from build123d import *

# Parameters (mm, degrees)
SKETCH1_W             = 35
SKETCH1_H             = 35
BOSS_EXTRUDE1_DEPTH   = 10
BOSS_EXTRUDE2_DEPTH   = 6
M10_CLEARANCE_HOLE1_D = 11
M6_CLEARANCE_HOLE1_D  = 6.6
MIRROR2_COPY_1_D      = 6.6


with BuildPart() as part:
    # Sketch1 → Boss-Extrude1 (new body)
    # profile 1 of 2: a face of its own
    with BuildSketch(Plane(origin=(0, 0, 0), x_dir=(1, 0, 0), z_dir=(0, 1, 0))):
        Rectangle(SKETCH1_W, SKETCH1_H)
        Polygon((-5.17766953, -12.5), (5.17766953, -12.5), (12.5, -5.17766953), (12.5, 5.17766953), (5.17766953, 12.5), (-5.17766953, 12.5), (-12.5, 5.17766953), (-12.5, -5.17766953), align=None, mode=Mode.SUBTRACT)
    # profile 2 of 2: a face of its own
    with BuildSketch(Plane(origin=(0, 0, 0), x_dir=(1, 0, 0), z_dir=(0, 1, 0))):
        Polygon((-12.5, -5.17766953), (-5.17766953, -12.5), (5.17766953, -12.5), (12.5, -5.17766953), (12.5, 5.17766953), (5.17766953, 12.5), (-5.17766953, 12.5), (-12.5, 5.17766953), align=None)
    extrude(amount=-BOSS_EXTRUDE1_DEPTH)

    # Sketch1_3 → Boss-Extrude2 (add)
    with BuildSketch(Plane(origin=(0, 0, 0), x_dir=(1, 0, 0), z_dir=(0, 1, 0))):
        Polygon((-12.5, -5.17766953), (-5.17766953, -12.5), (5.17766953, -12.5), (12.5, -5.17766953), (12.5, 5.17766953), (5.17766953, 12.5), (-5.17766953, 12.5), (-12.5, 5.17766953), align=None)
    extrude(amount=BOSS_EXTRUDE2_DEPTH)

    # M10 Clearance Hole1 (through all)
    with Locations(Plane(origin=(0, 6, 0), x_dir=(1, 0, 0), z_dir=(0, 1, 0))):
        with Locations((0, 0)):
            Hole(M10_CLEARANCE_HOLE1_D / 2)

    # M6 Clearance Hole1 (through all)
    with Locations(Plane(origin=(0, 0, 0), x_dir=(1, 0, 0), z_dir=(0, 1, 0))):
        with Locations((-12.5, 12.5)):
            m6_clearance_hole1 = Hole(M6_CLEARANCE_HOLE1_D / 2)

    # Mirror1: M6 Clearance Hole1 across plane
    add(m6_clearance_hole1.mirror(Plane(origin=(0, 0, 0), x_dir=(0, 0, 1), z_dir=(1, 0, 0))), mode=Mode.SUBTRACT)

    # Mirror2: M6 Clearance Hole1 across plane
    add(m6_clearance_hole1.mirror(Plane.XY), mode=Mode.SUBTRACT)

    # Mirror2 copy 1 (through all)
    with Locations(Plane(origin=(0, 0, 0), x_dir=(-1, 0, 0), z_dir=(0, 1, 0))):
        with Locations((-12.5, 12.5)):
            Hole(MIRROR2_COPY_1_D / 2)


solid = part.part
Can you work these out from the model? Positions are in its coordinate system, mm. A direction names the side the tool comes from. Coordinates: 2 decimals unless noted, no trailing zeros. Loops run counter-clockwise (first coordinate to the right, second up) from the corner with the lowest first, then second, coordinate; pieces in that order, holes last. Notation, with made-up numbers: (12.25, 55.25) - (26.25, 55.25) arc R26 cw to (26.25, 71.25) - close; hole circle Ø3 at (-13, -5). An arc over 180 degrees is marked (long way). Answer as a JSON object with one key per item and string values. Group by question number.
Item 1: If we mould it in two halves opening along Z, with no side actions, what happens to faces 6 (the face through (-9.881, -5.07, -10.492)), 7 (the face through (0, 3, -12.5)), 8 (the face through (8.79, 2.96, 8.89)), 9 (the face through (0, 6, -6))? For each: released by +Z, released by -Z, zero draft, split by the parting line, or undercut.
Item 2: If we section it at D-D (x = 11.5): List the corners of the cut face in (y, z) for me.
Item 3: For pin 1 (9 mm diameter, centred on x = 0, z = 0, fed in from -Y); pin 2 (7.5 mm diameter, centred on x = -12.5, z = -12.5, fed in from +Y); pin 3 (5 mm diameter, centred on y = 4, z = -1.5, fed in from +X); pin 4 (3 mm diameter, centred on x = -0.5, y = 4, fed in from +Z), each with a flat end and sliding along its axis, tell me the tip position at first contact or that it passes through.
Item 4: If we section it at B-B (x = -3): List the corners of the cut face in (y, z) for me.
Item 5: If we section it at A-A (z = 0): List the corners of the cut face in (x, y) for me.
Item 6: If I drill on L1, parallel to Z at x = -12.5, y = -4.5; L2, parallel to Z at x = 0, y = -5.25; L3, parallel to Z at x = 15.5, y = -6.5, over which ranges is the centre line in solid material (lowest first)? Write a range as from..to.
Item 7: If we section it at C-C (y = -1.5): List the corners of the cut face in (x, z) for me.
Item 8: On a 3-axis mill with a long thin cutter (end or side, diameter ignored), from which of +Z, -Z, +X, -X, +Y, -Y can I reach the whole of each face in a straight line? I mean faces 1 (the face through (8.89, 2.96, -8.79)), 2 (the face through (-8.89, 2.96, 8.79)), 3 (the face through (-12.5, 3, 0)), 4 (the face through (-8.79, 2.96, -8.89)), 5 (the face through (-12, 0, -8)). Say none if no direction works.
Returned:
{
 "1": {"face 6": "undercut", "face 7": "released by -Z", "face 8": "released by +Z", "face 9": "zero draft"},
 "2": {"outline": "(-10, -17.5) - (0, -17.5) - (0, -15.64) - (-10, -15.64) - close; (-10, -9.36) - (0, -9.36) - (0, -6.18) - (6, -6.18) - (6, 6.18) - (0, 6.18) - (0, 9.36) - (-10, 9.36) - close; (-10, 15.64) - (0, 15.64) - (0, 17.5) - (-10, 17.5) - close"},
 "3": {"pin 1": "passes through", "pin 2": "stops at y = 0", "pin 3": "stops at x = 12.5", "pin 4": "stops at z = 12.5"},
 "4": {"outline": "(-10, -17.5) - (0, -17.5) - (0, -12.5) - (6, -12.5) - (6, -4.61) - (-10, -4.61) - close; (-10, 4.61) - (6, 4.61) - (6, 12.5) - (0, 12.5) - (0, 17.5) - (-10, 17.5) - close"},
 "5": {"outline": "(-17.5, -10) - (-5.5, -10) - (-5.5, 6) - (-12.5, 6) - (-12.5, 0) - (-17.5, 0) - close; (5.5, -10) - (17.5, -10) - (17.5, 0) - (12.5, 0) - (12.5, 6) - (5.5, 6) - close"},
 "6": {"L1": "z = -17.5..-15.8, -9.2..9.2, 15.8..17.5", "L2": "z = -17.5..-5.5, 5.5..17.5", "L3": "z = -17.5..-13.87, -11.13..11.13, 13.87..17.5"},
 "7": {"outline": "(-17.5, -17.5) - (17.5, -17.5) - (17.5, 17.5) - (-17.5, 17.5) - close; hole circle Ø6.6 at (-12.5, -12.5); hole circle Ø6.6 at (-12.5, 12.5); hole circle Ø11 at (0, 0); hole circle Ø6.6 at (12.5, -12.5); hole circle Ø6.6 at (12.5, 12.5)"},
 "8": {"face 1": "-Z, +X, +Y", "face 2": "+Z, -X, +Y", "face 3": "+Z, -Z, -X, +Y", "face 4": "-Z, -X, +Y", "face 5": "+Y"}
}
